Read the model definition and answer for the solid it produces. Units are mm, in the model's axes. Give positions to 0.01 mm unless a question says otherwise; leave off trailing zeros. Write each loop counter-clockwise with the first axis right and the second up, starting at its lowest first coordinate (ties: lowest second). Pieces come first, ordered by that corner, then holes.
```python
from build123d import *

# Parameters (mm, degrees)
SKETCH_W     = 25
SKETCH_H     = 25
SKETCH_W_2   = 22
SKETCH_H_2   = 22
PAD_DEPTH    = 793
FILLET_R     = 0.74
POCKET_DEPTH = 25.001


with BuildPart() as part:
    # Sketch → Pad (new body)
    with BuildSketch(Plane.XY):
        with Locations((12.5, 12.5)):
            Rectangle(SKETCH_W, SKETCH_H)
        with Locations((12.5, 12.5)):
            Rectangle(SKETCH_W_2, SKETCH_H_2, mode=Mode.SUBTRACT)
    extrude(amount=PAD_DEPTH)

    # Fillet
    fillet_edges = [part.edges().sort_by_distance(p)[0] for p in [
        (25, 0, 396.5),
        (0, 0, 396.5),
        (25, 25, 396.5),
        (0, 25, 396.5),
    ]]
    fillet(fillet_edges, radius=FILLET_R)

    # Sketch001 (on Face6 of Fillet) → Pocket (cut, through all)
    with BuildSketch(Plane(origin=(0, 0, 0), x_dir=(0, -1, 0), z_dir=(-1, 0, 0))):
        Polygon((0, 0), (-33.812955, 117.919787), (-33.812955, -15.683764), align=None)
    extrude(amount=-POCKET_DEPTH, mode=Mode.SUBTRACT)


solid = part.part
```
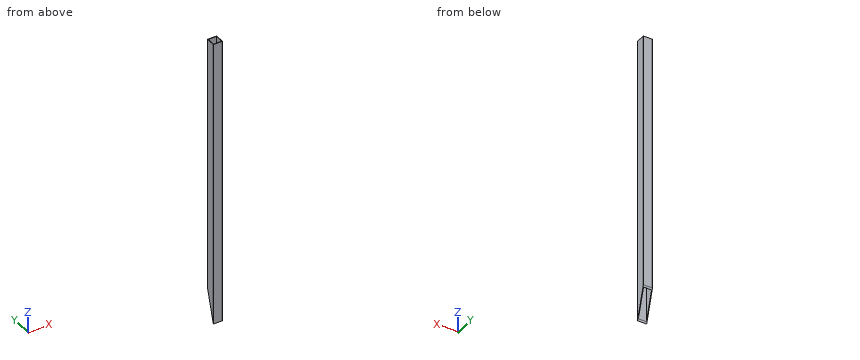
Item 1: Find the intervals of material crossed by line 1 along Y through (x, z) = (13, 302), in increasing order.
Result set:
line 1: y = 0 to 1.5, 23.5 to 25
Item 2: Section C-C (y = 13.25) is taken. Write down the section's boundary in (x, z), and give its area (3 significant figures).
Result set:
outline: (0, 46.21) - (1.5, 46.21) - (1.5, 793) - (0, 793) - close; (23.5, 46.21) - (25, 46.21) - (25, 793) - (23.5, 793) - close
area: 2,240 mm2
Item 3: Section A-A (x = 10.5) is taken. Write down the section's boundary in (y, z).
Result set:
outline: (0, 0) - (1.5, 5.23) - (1.5, 793) - (0, 793) - close; (23.5, 81.95) - (25, 87.19) - (25, 793) - (23.5, 793) - close
Item 4: Section B-B (z = 470) is taken. Write down the section's boundary in (x, y).
Result set:
outline: (0, 0.74) arc R0.74 ccw to (0.74, 0) - (24.26, 0) arc R0.74 ccw to (25, 0.74) - (25, 24.26) arc R0.74 ccw to (24.26, 25) - (0.74, 25) arc R0.74 ccw to (0, 24.26) - close; hole (1.5, 1.5) - (23.5, 1.5) - (23.5, 23.5) - (1.5, 23.5) - close
